Autodesk Fusion 360 part; units mm, degrees
sketch "Base" plane through (0, 0, 0) normal (0, 1, 0) x (1, 0, 0) in component "Squeegee Holder"
  line L0 (4.4321, 10.7) -> (-4.4321, 10.7)
  line L1 (-4.4321, 10.7) -> (-10.7, 4.4321)
  line L2 (-10.7, 4.4321) -> (-10.7, -4.4321)
  line L3 (-10.7, -4.4321) -> (-4.4321, -10.7)
  line L4 (-4.4321, -10.7) -> (4.4321, -10.7)
  line L5 (4.4321, -10.7) -> (10.7, -4.4321)
  line L6 (10.7, -4.4321) -> (10.7, 4.4321)
  line L7 (10.7, 4.4321) -> (4.4321, 10.7)
  line L8 (10.65, 4.4114) -> (4.4114, 10.65)
  line L9 (4.4114, 10.65) -> (-4.4114, 10.65)
  line L10 (-4.4114, 10.65) -> (-10.65, 4.4114)
  line L11 (-10.65, 4.4114) -> (-10.65, -4.4114)
  line L12 (-10.65, -4.4114) -> (-4.4114, -10.65)
  line L13 (-4.4114, -10.65) -> (4.4114, -10.65)
  line L14 (4.4114, -10.65) -> (10.65, -4.4114)
  line L15 (10.65, -4.4114) -> (10.65, 4.4114)
  line L16 (12.5, 5.1777) -> (5.1777, 12.5)
  line L17 (5.1777, 12.5) -> (-5.1777, 12.5)
  line L18 (-5.1777, 12.5) -> (-12.5, 5.1777)
  line L19 (-12.5, 5.1777) -> (-12.5, -5.1777)
  line L20 (-12.5, -5.1777) -> (-5.1777, -12.5)
  line L21 (-5.1777, -12.5) -> (5.1777, -12.5)
  line L22 (5.1777, -12.5) -> (12.5, -5.1777)
  line L23 (12.5, -5.1777) -> (12.5, 5.1777)
  line L24 (6.75, 2.7959) -> (2.7959, 6.75)
  line L25 (2.7959, 6.75) -> (-2.7959, 6.75)
  line L26 (-2.7959, 6.75) -> (-6.75, 2.7959)
  line L27 (-6.75, 2.7959) -> (-6.75, -2.7959)
  line L28 (-6.75, -2.7959) -> (-2.7959, -6.75)
  line L29 (-2.7959, -6.75) -> (2.7959, -6.75)
  line L30 (2.7959, -6.75) -> (6.75, -2.7959)
  line L31 (6.75, -2.7959) -> (6.75, 2.7959)
  line L32 (-4.9706, 12) -> (-12, 4.9706)
  line L33 (-12, 4.9706) -> (-12, -4.9706)
  line L34 (-12, -4.9706) -> (-4.9706, -12)
  line L35 (-4.9706, -12) -> (4.9706, -12)
  line L36 (4.9706, -12) -> (12, -4.9706)
  line L37 (12, -4.9706) -> (12, 4.9706)
  line L38 (12, 4.9706) -> (4.9706, 12)
  line L39 (4.9706, 12) -> (-4.9706, 12)
  dimension "d4" = 21.4
  dimension "d5" = 25
  dimension "d56" = 13.5
  dimension "d66" = 24
sketch "Notch" plane through (0, 0, 0) normal (0, 1, 0) x (1, 0, 0) in component "Squeegee Holder"
  line L0 (-4.4114, -10.65) -> (4.4114, -10.65) construction
  line L1 (3, -6.75) -> (-3, -6.75) construction
  line L2 (-3, -6.75) -> (-3, -9.75)
  line L3 (-3, -9.75) -> (3, -9.75)
  line L4 (3, -9.75) -> (3, -6.75)
  line L5 (-3, -6.75) -> (-3, -6.25)
  line L6 (3, -6.75) -> (3, -6.25)
  line L7 (3, -6.25) -> (-3, -6.25)
  line L8 (3, 9.75) -> (-3, 9.75)
  line L9 (-3, 9.75) -> (-3, 6.75)
  line L10 (3, 6.75) -> (3, 9.75)
  line L11 (3, 6.75) -> (3, 6.25)
  line L12 (-3, 6.75) -> (-3, 6.25)
  line L13 (-3, 6.25) -> (3, 6.25)
  line L14 (-2.7959, -6.75) -> (2.7959, -6.75)
  dimension "d24" = 6
  dimension "d25" = 3
  dimension "d31" = 360
  dimension "d57" = 0.5
extrude "Extrude5" add sketch "Base" along normal blind 6.4 contours L8 L9 L10 L11 L12 L13 L14 L15 | L24 L25 L26 L27 L28 L29 L30 L31 in component "Squeegee Holder"
extrude "Extrude10" add sketch "Base" against normal blind 2.6 contours L0 L1 L2 L3 L4 L5 L6 L7 | L8 L9 L10 L11 L12 L13 L14 L15 | L16 L17 L18 L19 L20 L21 L22 L23 | L24 L25 L26 L27 L28 L29 L30 L31 | L32 L33 L34 L35 L36 L37 L38 L39 in component "Squeegee Holder"
extrude "Extrude6" cut sketch "Base" along normal through all and the other way through all contours L24 L25 L26 L27 L28 L29 L30 L31 in component "Squeegee Holder"
extrude "Extrude8" cut sketch "Notch" against normal blind 3.6 from surface at 6.4 in component "Squeegee Holder"
sketch "Marca" plane through (0, -2.6, 0) normal (0, 1, 0) x (1, 0, 0) in component "Squeegee Holder"
  circle A0 centre (0, -9.625) radius 1
  line L0 (-2.7959, 6.75) -> (-6.75, 2.7959)
  line L1 (-6.75, 2.7959) -> (-6.75, -2.7959)
  line L2 (-6.75, -2.7959) -> (-2.7959, -6.75)
  line L3 (-2.7959, -6.75) -> (2.7959, -6.75)
  line L4 (2.7959, -6.75) -> (6.75, -2.7959)
  line L5 (6.75, -2.7959) -> (6.75, 2.7959)
  line L6 (6.75, 2.7959) -> (2.7959, 6.75)
  line L7 (2.7959, 6.75) -> (-2.7959, 6.75)
  line L8 (12.5, 5.1777) -> (12.5, -5.1777)
  line L9 (12.5, -5.1777) -> (5.1777, -12.5)
  line L10 (5.1777, -12.5) -> (-5.1777, -12.5)
  line L11 (-5.1777, -12.5) -> (-12.5, -5.1777)
  line L12 (-12.5, -5.1777) -> (-12.5, 5.1777)
  line L13 (-12.5, 5.1777) -> (-5.1777, 12.5)
  line L14 (-5.1777, 12.5) -> (5.1777, 12.5)
  line L15 (5.1777, 12.5) -> (12.5, 5.1777)
  line L16 (0, -12.5) -> (0, -6.75) construction
  dimension "d61" = 2
extrude "Extrude9" cut sketch "Marca" along normal blind 0.4 contours A0 in component "Squeegee Holder"
chamfer "Chamfer3" distance 0.6 angle 45 32 edges at (0, 6.4, 10.65) (7.5307, 6.4, 7.5307) (10.65, 6.4, 0) (7.5307, 6.4, -7.5307) (0, 6.4, -10.65) (-7.5307, 6.4, -7.5307) (-10.65, 6.4, 0) (-7.5307, 6.4, 7.5307) (12.5, 0, 0) (8.8388, 0, 8.8388) (8.8388, -2.6, 8.8388) (12.5, -2.6, 0) (0, 0, 12.5) (0, -2.6, 12.5) (8.8388, 0, -8.8388) (8.8388, -2.6, -8.8388) (0, -2.6, -12.5) (0, 0, -12.5) (-8.8388, 0, -8.8388) (-8.8388, -2.6, -8.8388) (-12.5, -2.6, 0) (-12.5, 0, 0) (-8.8388, 0, 8.8388) (-8.8388, -2.6, 8.8388) (0, -2.6, 6.75) (4.773, -2.6, 4.773) (6.75, -2.6, 0) (4.773, -2.6, -4.773) (0, -2.6, -6.75) (-4.773, -2.6, -4.773) (-6.75, -2.6, 0) (-4.773, -2.6, 4.773) in component "Squeegee Holder"
component "Squeegee Holder" placed x (1, 0, 0) y (0, 1, 0) z (0, 0, 1) at (0, 0, 0)
equation "d31 = C-Pattern1-Angle"
equation "Clearance_Tight = 0.05 mm"
Check sheet for the modelled part. Datum: model origin and axes. Units: mm. A direction names the side the tool comes from. Round coordinates to 2 decimals unless told otherwise and drop trailing zeros. Loops run counter-clockwise (first coordinate to the right, second up) from the corner with the lowest first, then second, coordinate; pieces in that order, holes last.
1. Sectioned sample at D-D on x = 9.25. Record the boundary of the cut face in (y, z).
2. Sectioned sample at B-B on x = 0. Record the boundary of the cut face in (y, z) (3 decimals).
3. Scan lines: probe 1 along X at (y, z) = (3.5, 3); probe 2 along Z at (x, y) = (2.5, 5.25); probe 3 along Z at (x, y) = (0, -2.25) (3 decimals). Record each from-to range of solid material in increasing order.
4. Mould release check, pull along Z, two halves, no side actions. Record for faces 5 (the flat face through (-8.89, -1.29, 8.79)), 6 (the flat face through (3, 5, 8)), 7 (the flat face through (-8.681, -0.304, -8.578)): released by +Z, released by -Z, zero draft, split by the parting line, or undercut.
5. Sectioned sample at A-A on z = -2.5. Record the boundary of the cut face in (x, y), and give its area (3 significant figures).
6. Gauge pin test, flat ends, axial feed: pin 1 Ø3 at (x, y) = (9, -1) entering from +Z; pin 2 Ø3.5 at (y, z) = (5, 8.5) entering from -X; pin 3 Ø3.5 at (y, z) = (5, -8) entering from -X. Record the tip position at first contact, or that the pin passes through.
7. Sectioned sample at C-C on y = 2. Record the boundary of the cut face in (x, z), and give its area (3 significant figures).
8. Set-up check for faces 1 (the flat face through (5.012, -2.296, -4.952)), 2 (the flat face through (-7.49, 2.86, -7.57)), 3 (the flat face through (0, 2.8, -9)), 4 (the flat face through (6.75, 2, 0)): record each of +Z, -Z, +X, -X, +Y, -Y from which the full face is reachable in a straight line by a thin tool's end or side.
Recorded:
1. outline: (-2.6, -7.58) - (-2, -8.43) - (-0.6, -8.43) - (0, -7.58) - (0, -5.81) - (5.8, -5.81) - (6.4, -4.96) - (6.4, 4.96) - (5.8, 5.81) - (0, 5.81) - (0, 7.58) - (-0.6, 8.43) - (-2, 8.43) - (-2.6, 7.58) - close
2. outline: (-2.6, -11.9) - (-2, -12.5) - (-0.6, -12.5) - (0, -11.9) - (0, -10.65) - (5.8, -10.65) - (6.4, -10.05) - (6.4, -9.75) - (2.8, -9.75) - (2.8, -6.75) - (-2, -6.75) - (-2.6, -7.35) - close; (-2.6, 7.35) - (-2, 6.75) - (2.8, 6.75) - (2.8, 9.75) - (6.4, 9.75) - (6.4, 10.05) - (5.8, 10.65) - (0, 10.65) - (0, 11.9) - (-0.6, 12.5) - (-2, 12.5) - (-2.6, 11.9) - (-2.6, 10.625) - (-2.2, 10.625) - (-2.2, 8.625) - (-2.6, 8.625) - close
3. probe 1: x = -10.65 to -6.55, 6.55 to 10.65
3. probe 2: z = -10.65 to -9.75, 9.75 to 10.65
3. probe 3: z = -12.25 to -7, 7 to 8.625, 10.625 to 12.25
4. face 5: released by +Z
4. face 6: undercut
4. face 7: released by -Z
5. outline: (-12.5, -2) - (-11.9, -2.6) - (-7.35, -2.6) - (-6.75, -2) - (-6.75, 6.4) - (-10.05, 6.4) - (-10.65, 5.8) - (-10.65, 0) - (-11.9, 0) - (-12.5, -0.6) - close; (6.75, -2) - (7.35, -2.6) - (11.9, -2.6) - (12.5, -2) - (12.5, -0.6) - (11.9, 0) - (10.65, 0) - (10.65, 5.8) - (10.05, 6.4) - (6.75, 6.4) - close
5. area: 78.4 mm2
6. pin 1: stops at z = 10.18
6. pin 2: stops at x = -8.31
6. pin 3: stops at x = -8.81
7. outline: (-10.65, -4.41) - (-4.41, -10.65) - (4.41, -10.65) - (10.65, -4.41) - (10.65, 4.41) - (4.41, 10.65) - (-4.41, 10.65) - (-10.65, 4.41) - close; hole (-6.75, -2.8) - (-2.8, -6.75) - (2.8, -6.75) - (6.75, -2.8) - (6.75, 2.8) - (2.8, 6.75) - (-2.8, 6.75) - (-6.75, 2.8) - close
7. area: 225 mm2
8. face 1: -Y
8. face 2: -Z, -X, +Y
8. face 3: +Y
8. face 4: +Y, -Y
